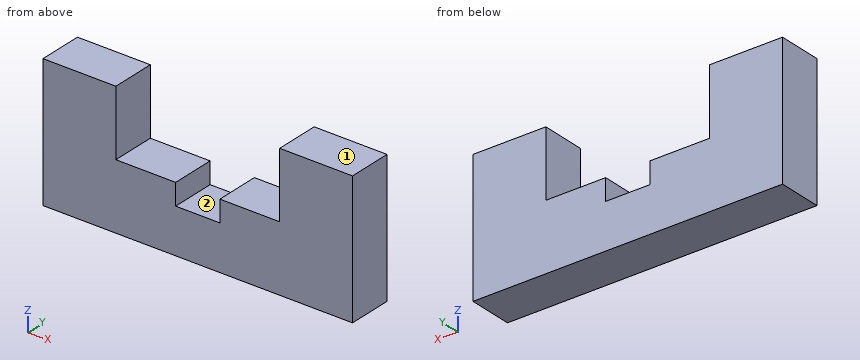
from build123d import *

# Parameters (mm, degrees)
F1_DEPTH = 25.4
F2_W     = 25.4
F2_H     = 12.321454
F3_DEPTH = 4
F4_DEPTH = 25.401


with BuildPart() as f1:
    # F0 (on Front) → F1 (new body)
    with BuildSketch(Plane.XZ):
        Polygon((-47.05, 25.021454), (-88.9, 25.021454), (-88.9, -30.673691), (-88.9, -51.178546), (-41.565981, -51.178546), (0, -51.178546), (88.9, -51.178546), (88.9, 25.021454), (47.05, 25.021454), (47.05, -13.078546), (0, -13.078546), (-47.05, -13.078546), align=None)
    extrude(amount=F1_DEPTH)

    # F2 (on Front) → F3 (cut)
    with BuildSketch(Plane.XZ):
        with Locations((0, -19.239273)):
            Rectangle(F2_W, F2_H)
    extrude(amount=F3_DEPTH, mode=Mode.SUBTRACT)

    # F2 (on Front) → F4 (cut, through all)
    with BuildSketch(Plane.XZ):
        with Locations((0, -19.239273)):
            Rectangle(F2_W, F2_H)
    extrude(amount=F4_DEPTH, mode=Mode.SUBTRACT)


solid = f1.part
Here's how the part is built. I have some questions about the finished solid (model axes, mm). Face numbers are marked on the shaded views. A direction names the side the tool comes from. Round coordinates to 2 decimals unless told otherwise and drop trailing zeros. Write each loop counter-clockwise with the first axis right and the second up, starting at its lowest first coordinate (ties: lowest second). Pieces come first, ordered by that corner, then holes.
1. Will this pin go through, and if not, where does the flat tip stop? pin 1 Ø7.5 at (x, y) = (28.5, -8.5) entering from +Z.
2. Suppose I cut it at B-B (y = -13.5). List the corners of the cut face in (x, z) for me, and give its area (3 significant figures).
3. For the marked faces 1 and 2, which set-ups out of +Z, -Z, +X, -X, +Y, -Y let a thin tool reach every point of the face, with its end or its side?
4. Suppose I cut it at C-C (x = 8.5). List the corners of the cut face in (y, z) for me.
5. Suppose I cut it at D-D (x = -20). List the corners of the cut face in (y, z) for me.
6. I need wall thicknesses on L1, parallel to X at y = -16.75, z = 10; L2, parallel to Z at x = 29.5, y = -7.25; L3, parallel to Z at x = 6.5, y = -14.75. Which ranges of each line are inside material? Lowest first, please.
7. Suppose I cut it at A-A (z = -11). List the corners of the cut face in (x, y) for me, and give its area (3 significant figures).
Answer sheet:
1. pin 1: stops at z = -13.08
2. outline: (-88.9, -51.18) - (88.9, -51.18) - (88.9, 25.02) - (47.05, 25.02) - (47.05, -13.08) - (12.7, -13.08) - (12.7, -25.4) - (-12.7, -25.4) - (-12.7, -13.08) - (-47.05, -13.08) - (-47.05, 25.02) - (-88.9, 25.02) - close
2. area: 9,650 mm2
3. face 1: +Z, +X, -X, +Y, -Y
3. face 2: +Z, +Y, -Y
4. outline: (-25.4, -51.18) - (0, -51.18) - (0, -25.4) - (-25.4, -25.4) - close
5. outline: (-25.4, -51.18) - (0, -51.18) - (0, -13.08) - (-25.4, -13.08) - close
6. L1: x = -88.9 to -47.05, 47.05 to 88.9
6. L2: z = -51.18 to -13.08
6. L3: z = -51.18 to -25.4
7. outline: (-88.9, -25.4) - (-47.05, -25.4) - (-47.05, 0) - (-88.9, 0) - close; (47.05, -25.4) - (88.9, -25.4) - (88.9, 0) - (47.05, 0) - close
7. area: 2,130 mm2
